Design review of the part built by this model. Coordinates are the model's own, in mm. A direction names the side the tool comes from. Round coordinates to 2 decimals unless told otherwise and drop trailing zeros. Loops run counter-clockwise (first coordinate to the right, second up) from the corner with the lowest first, then second, coordinate; pieces in that order, holes last. Notation, with made-up numbers: M 44,-12.5 L 83,-12.5 A28 ccw 83,17.5 Z; hole C -8.5,70.25 d4. An arc over 180 degrees is marked long. One line per item, written item: value. Start each with the question number.
Item 1: We need section B-B (x = -51). Write out the cut boundary in (y, z), then the cut area to 3 significant figures.
Item 2: Clearance check with flat-ended pins moving along their axes: pin 1 (1.8 mm diameter, centred on y = -4, z = 1, fed in from +X); pin 2 (1.2 mm diameter, centred on x = -32.5, y = -5.5, fed in from -Z); pin 3 (6 mm diameter, centred on y = -3, z = 1, fed in from +X); pin 4 (3 mm diameter, centred on x = 0, y = -5, fed in from -Z). State where each tip first meets the part, or that it passes through.
Item 3: We need section A-A (x = 0). Write out the cut boundary in (y, z), then the cut area to 3 significant figures.
Item 4: For line 1 along Z through (x, y) = (42, -5.25); line 2 along X through (y, z) = (-1.75, 0.25); line 3 along Z through (x, y) = (8, -3.75), list the stretches that pass through material, from the lowest coordinate up.
Item 5: Mouldability with a two-part tool opening along Z and no side actions: class faces 1 (the flat face through (-2, -10, 2)), 2 (the flat face through (-32, -5, 0)), 3 (the flat face through (41, -5, -5)) as released by +Z, released by -Z, zero draft, split by the parting line, or undercut.
Item 6: We need section D-D (x = -18.5). Write out the cut boundary in (y, z).
Item 7: For faces 4 (the flat face through (-42.3, -1.5, -4)), 5 (the flat face through (-41, -5, 5)), 6 (the flat face through (-42.3, -8.5, -4)), 7 (the flat face through (42, -5, 5)), 8 (the cylindrical face through (51.8, -2.6, -1.8)), list the 3-axis set-ups (+Z, -Z, +X, -X, +Y, -Y) from which the entire face can be reached by the end or side of a thin tool; tool diameter is ignored.
Item 8: We need section C-C (y = -5). State how many separate pieces and enclosed holes the cut face has, then the cut area to 3 significant figures.
from build123d import *

# Parameters (mm, degrees)
F0_R          = 2
F0_R_2        = 0.5
F1_DEPTH      = 10
F2_R          = 3
F3_DEPTH      = 40
F4_R          = 1.75
F5_DEPTH      = 9.001
F5_DEPTH_BACK = 9.001
F6_R          = 10
F7_SIZE2      = 3
F7_SIZE       = 2
F7_2_SIZE2    = 3
F7_2_SIZE     = 2


# Not quite as in the source:
# - a pattern or mirror of a feature is missing from the dataset's text; its kind, count and spacing are read off the source's solid


with BuildPart() as f1:
    # F0 (on Front) → F1 (new body)
    with BuildSketch(Plane.XZ):
        with BuildLine():
            Line((71, 5), (7.4833147735, 5))
            ThreePointArc((7.4833147735, 5), (0, 9), (-7.4833147735, 5))
            Line((-7.4833147735, 5), (-72, 5))
            Line((-72, 5), (-72, -5))
            Line((-72, -5), (-7.4833147735, -5))
            ThreePointArc((-7.4833147735, -5), (0, -9), (7.4833147735, -5))
            Line((7.4833147735, -5), (71, -5))
            Line((71, -5), (71, 5))
        make_face()
        Circle(F0_R, mode=Mode.SUBTRACT)
        with Locations((8, 0)):
            Circle(F0_R_2, mode=Mode.SUBTRACT)
    extrude(amount=F1_DEPTH)

    # F2 (on face) → F3 (cut)
    with BuildSketch(Plane(origin=(-72, 0, 0), x_dir=(0, -1, 0), z_dir=(-1, 0, 0))):
        with Locations((5, 0)):
            Circle(F2_R)
    f3 = extrude(amount=-F3_DEPTH, mode=Mode.SUBTRACT)

    # F3_copies: F3 across plane
    add(f3.mirror(Plane(origin=(0, 0, 0), x_dir=(0, 0, 1), z_dir=(1, 0, 0))), mode=Mode.SUBTRACT)

    # F4 (on Top) → F5 (cut, two sides)
    with BuildSketch(Plane.XY) as f5_sk:
        with Locations((0, -5)):
            Circle(F4_R)
    extrude(amount=-F5_DEPTH, mode=Mode.SUBTRACT)
    extrude(f5_sk.sketch, amount=F5_DEPTH_BACK, mode=Mode.SUBTRACT)

    # F6
    f6_edges = [f1.edges().sort_by_distance(p)[0] for p in [
        (-7.483315, -5, 5),
        (7.483315, -5, 5),
        (7.483315, -5, -5),
        (-7.483315, -5, -5),
    ]]
    fillet(f6_edges, radius=F6_R)

    # F7
    f7_edges = [f1.edges().sort_by_distance(p)[0] for p in [
        (-41.830952, -10, 5),
        (-41.830952, -10, -5),
    ]]
    f7_side = f1.faces().sort_by_distance((41.330952, -10, -3.558716))[0]
    chamfer(f7_edges, length=F7_SIZE, length2=F7_SIZE2, reference=f7_side)

    # F7#2
    f7_2_edges = [f1.edges().sort_by_distance(p)[0] for p in [
        (-41.830952, 0, 5),
        (-41.830952, 0, -5),
    ]]
    f7_2_side = f1.faces().sort_by_distance((41.330952, 0, -3.558716))[0]
    chamfer(f7_2_edges, length=F7_2_SIZE, length2=F7_2_SIZE2, reference=f7_2_side)


solid = f1.part
A:
1. outline: M -10,-3 L -7,-5 L -3,-5 L 0,-3 L 0,3 L -3,5 L -7,5 L -10,3 Z; hole C -5,0 d6
1. area: 59.7 mm2
2. pin 1: x = 32
2. pin 2: z = -5
2. pin 3: x = 71
2. pin 4: through
3. outline: M -10,-7 L -7,-9 L -6.75,-9 L -6.75,-2 L -10,-2 Z; M -10,2 L -6.75,2 L -6.75,9 L -7,9 L -10,7 Z; M -3.25,-9 L -3,-9 L 0,-7 L 0,-2 L -3.25,-2 Z; M -3.25,2 L 0,2 L 0,7 L -3,9 L -3.25,9 Z
3. area: 79.0 mm2
4. line 1: -5 to -2.99, 2.99 to 5
4. line 2: -72 to -1.98, 1.98 to 7.57, 8.43 to 71
4. line 3: -5.69 to -0.5, 0.5 to 5.69
5. face 1: zero draft
5. face 2: undercut
5. face 3: released by -Z
6. outline: M -10,-3 L -7,-5 L -3,-5 L 0,-3 L 0,3 L -3,5 L -7,5 L -10,3 Z
7. face 4: -Z, -X, +Y
7. face 5: +Z, -X, +Y, -Y
7. face 6: -Z, -X, -Y
7. face 7: +Z, +X, +Y, -Y
7. face 8: +X
8. separate pieces: 2
8. enclosed holes: 1
8. area: 983 mm2
